For this review, take the finished solid that the model builds, in its own axes (mm). A direction names the side the tool comes from. Give positions to 0.01 mm unless a question says otherwise; leave off trailing zeros. Write each loop counter-clockwise with the first axis right and the second up, starting at its lowest first coordinate (ties: lowest second). Pieces come first, ordered by that corner, then holes. Notation, with made-up numbers: (-6.5, 3.25) -> (40.5, 3.25) arc R11 cw to (40.5, 16.25) -> close; hole circle Ø5 at (-23.5, -21.75). An arc over 180 degrees is marked (long way). Return JSON: item names as keys, results as strings.
Autodesk Inventor part; units mm, degrees
ref_plane "YZ Plane" through (0, 0, 0) normal (1, 0, 0) x (0, 1, 0)
ref_plane "XZ Plane" through (0, 0, 0) normal (0, 1, 0) x (-1, 0, 0)
ref_plane "XY Plane" through (0, 0, 0) normal (0, 0, 1) x (1, 0, 0)
sketch "Skizze1" plane through (0, 0, 0) normal (0, 1, 0) x (-1, 0, 0)
  line L0 (6.5, 0) -> (-6.5, 0)
  line L1 (-6.5, 0) -> (-6.5, 43)
  arc A0 (6.5, 43) -> (-6.5, 43) centre (0, 43) ccw
  line L2 (6.5, 43) -> (6.5, 0)
  line L3 (0, 0) -> (0, 43) construction
  point P0 (0, 0)
  dimension "d0" = 13
  dimension "d1" = 43
  dimension "d2" = 6.5
  dimension "d3" = 6.5
extrude "Extrusion1" add sketch "Skizze1" along normal blind 13
sketch "Skizze2" plane through (0, 13, 0) normal (0, 1, 0) x (1, 0, 0)
  arc A0 (-6.5, -43) -> (6.5, -43) centre (0, -43) ccw
  point P0 (0, 0)
hole "Bohrung1" at (0, 13, 43) direction (0, -1, 0) diameter 6 depth 13
sketch "Skizze3" plane through (6.5, 0, 0) normal (0, 0, -1) x (-1, 0, 0)
  circle A0 centre (6.5, 6.5) radius 3.5
  line L0 (0, 0) -> (0, 13)
  line L1 (0, 0) -> (13, 0)
  point P0 (6.5, 0)
  point P1 (0, 6.5)
  point P2 (6.5, 0)
  dimension "d13" = 7
extrude "Extrusion2" cut sketch "Skizze3" against normal blind 36
sketch "Skizze4" plane through (0, 0, 0) normal (0, -1, 0) x (1, 0, 0)
  circle A0 centre (0, 43) radius 3
  point P0 (0, 0)
  point P1 (0, 28.7)
  dimension "d23" = 14.3
hole "Bohrung2" at (0, 0, 28.7) direction (0, 1, 0) diameter 2 depth 4
properties part number "adapter" material "Aluminium 6061"
1. For pin 1 (2 mm diameter, centred on x = 0.5, y = 10, fed in from +Z); pin 2 (2 mm diameter, centred on x = 1.5, y = 7, fed in from -Z), all flat-tipped, find the tip position at first contact; note any pin that passes through.
Results found:
{"pin 1": "stops at z = 49.5", "pin 2": "stops at z = 36"}
2. The part is to be moulded in two halves that separate along Y. For faces 1 (the flat face through (0, 13, 25)), 2 (the flat face through (0, 7, 36)), 3 (the flat face through (-3, 9, 0)), say which applies: +Y half, -Y half, draft (parallel to the pull), parting line (faces both ways), or undercut.
Results found:
{"face 1": "+Y half", "face 2": "undercut", "face 3": "draft"}
3. To check wall thickness, follow probe 1 along Z at (x, y) = (0, 1.15); probe 2 along Z at (x, y) = (0, 9); probe 3 along X at (y, z) = (5.5, 43). State the ranges of each line that lie inside material, in increasing order.
Results found:
{"probe 1": "z = 0 to 27.7, 29.7 to 40, 46 to 49.5", "probe 2": "z = 36 to 40, 46 to 49.5", "probe 3": "x = -6.5 to -3, 3 to 6.5"}
4. Add section A-A, the plane x = 0. State the section outline as (y, z) points.
Results found:
{"outline": "(0, 0) -> (3, 0) -> (3, 27.7) -> (0, 27.7) -> close; (0, 29.7) -> (3, 29.7) -> (3, 36) -> (10, 36) -> (10, 0) -> (13, 0) -> (13, 40) -> (0, 40) -> close; (0, 46) -> (13, 46) -> (13, 49.5) -> (0, 49.5) -> close"}
5. Add section B-B, the plane y = 6.5. State the section outline as (x, z) points, plus the area to 3 significant figures.
Results found:
{"outline": "(-6.5, 0) -> (-3.5, 0) -> (-3.5, 36) -> (3.5, 36) -> (3.5, 0) -> (6.5, 0) -> (6.5, 43) arc R6.5 ccw to (-6.5, 43) -> close; hole circle Ø6 at (0, 43)", "area": "345 mm²"}
6. Add section C-C, the plane z = 8. State the section outline as (x, y) points, plus the area to 3 significant figures.
Results found:
{"outline": "(-6.5, 0) -> (6.5, 0) -> (6.5, 13) -> (-6.5, 13) -> close; hole circle Ø7 at (0, 6.5)", "area": "131 mm²"}
7. For faces 4 (the cylindrical face through (0.759, 3.083, 17.748)), 5 (the cylindrical face through (0, 6, 40)), 6 (the cylindrical face through (0, 1.6, 29.7)), list the 3-axis set-ups (+Z, -Z, +X, -X, +Y, -Y) from which the entire face can be reached by the end or side of a thin tool; tool diameter is ignored.
Results found:
{"face 4": "-Z", "face 5": "+Y, -Y", "face 6": "-Y"}
8. Add section D-D, the plane z = 42.5. State the section outline as (x, y) points, plus the area to 3 significant figures.
Results found:
{"outline": "(-6.5, 0) -> (-2.96, 0) -> (-2.96, 13) -> (-6.5, 13) -> close; (2.96, 0) -> (6.5, 0) -> (6.5, 13) -> (2.96, 13) -> close", "area": "92.1 mm²"}
